Check sheet for the modelled part. Datum: model origin and axes. Units: mm. A direction names the side the tool comes from. Give positions to 0.01 mm unless a question says otherwise; leave off trailing zeros. Loops run counter-clockwise (first coordinate to the right, second up) from the corner with the lowest first, then second, coordinate; pieces in that order, holes last. Notation, with made-up numbers: M -35,-39 L -8,-39 A29 cw -8,-1 Z; hole C 33.25,-19.5 d8. An arc over 180 degrees is marked long. Use one line per item in the form item = value.
from build123d import *

# Parameters (mm, degrees)
F0_R     = 76.2
F3_T     = -6.35
F0_R_2   = 95.25
F4_DEPTH = 12.7
F6_R     = 95.25
F6_R_2   = 76.2
F7_DEPTH = 12.7


with BuildPart() as f2:
    # F2: sweep along a path in F1
    with BuildLine(Plane.XY) as f2_path:
        Line((0, 0), (0, 152.4))
        ThreePointArc((0, 152.4), (44.6369265472, 260.1630734528), (152.4, 304.8))
        Line((152.4, 304.8), (304.8, 304.8))
    # F0 (on Front) → F2 (sweep)
    with BuildSketch(Plane.XZ):
        Circle(F0_R)
    sweep(path=f2_path.line)

    # F3
    f3_openings = [f2.faces().sort_by_distance(p)[0] for p in [
        (0, 0, 0),
        (304.8, 304.8, 0),
    ]]
    offset(amount=F3_T, openings=f3_openings)

    # F0 (on Front) → F4 (join)
    with BuildSketch(Plane.XZ):
        Circle(F0_R_2)
        Circle(F0_R, mode=Mode.SUBTRACT)
    extrude(amount=-F4_DEPTH)

    # F6 (on line) → F7 (join)
    with BuildSketch(Plane.YZ.offset(304.8)):
        with Locations((304.8, 0)):
            Circle(F6_R)
        with Locations((304.8, 0)):
            Circle(F6_R_2, mode=Mode.SUBTRACT)
    extrude(amount=-F7_DEPTH)


solid = f2.part
1) Depth check by flat-ended pin: pin 1 Ø3 at (y, z) = (249, -32.5) entering from -X; pin 2 Ø5 at (y, z) = (101.5, 27) entering from -X; pin 3 Ø12 at (x, z) = (28.5, 31.5) entering from +Y. Enter the tip coordinate at first touch or a pass-through.
Evaluation:
pin_1 = -47.78
pin_2 = -72.15
pin_3 = 341.3
2) Scan lines: line 1 (Z direction, x = 237, y = 304.8); line 2 (X direction, y = 146, z = -17); line 3 (Y direction, x = 264, z = 30). Record each from-to range of solid material in increasing order.
Evaluation:
line_1 = -76.2 to -69.85, 69.85 to 76.2
line_2 = -74.28 to -67.75, 67.75 to 74.28
line_3 = 234.75 to 241.72, 367.88 to 374.85
3) Section check C-C (z = -82). Record the cut outline in (x, y).
Evaluation:
outline = M -48.46,0 L 48.46,0 L 48.46,12.7 L -48.46,12.7 Z; M 292.1,256.34 L 304.8,256.34 L 304.8,353.26 L 292.1,353.26 Z
4) Release check for a two-part mould opening along Y. For faces 4 (the face through (223.23, 232.12, -22.89)), 5 (the face through (-55.431, 77.267, 42.503)), 6 (the face through (-60.47, 83.528, 46.367)) record: pulls with the +Y half, pulls with the -Y half, needs draft (parallel to the pull), parting line crosses it, or undercut.
Evaluation:
face_4 = parting line crosses it
face_5 = needs draft
face_6 = undercut
5) Section check A-A (z = 0). Record the cut outline in (x, y), then the cut area to 3 significant figures.
Evaluation:
outline = M -95.25,0 L -69.85,0 L -69.85,152.4 A222.25 cw 152.4,374.65 L 304.8,374.65 L 304.8,400.05 L 292.1,400.05 L 292.1,381 L 152.4,381 A228.6 ccw -76.2,152.4 L -76.2,12.7 L -95.25,12.7 Z; M 69.85,0 L 95.25,0 L 95.25,12.7 L 76.2,12.7 L 76.2,152.4 A76.2 cw 152.4,228.6 L 292.1,228.6 L 292.1,209.55 L 304.8,209.55 L 304.8,234.95 L 152.4,234.95 A82.55 ccw 69.85,152.4 Z
area = 7,880 mm^2
6) Section check D-D (z = -27.5). Record the cut outline in (x, y), then the cut area to 3 significant figures.
Evaluation:
outline = M -91.19,0 L -64.21,0 L -64.21,152.4 A216.61 cw 152.4,369.01 L 304.8,369.01 L 304.8,395.99 L 292.1,395.99 L 292.1,375.86 L 152.4,375.86 A223.46 ccw -71.06,152.4 L -71.06,12.7 L -91.19,12.7 Z; M 64.21,0 L 91.19,0 L 91.19,12.7 L 71.06,12.7 L 71.06,152.4 A81.34 cw 152.4,233.74 L 292.1,233.74 L 292.1,213.61 L 304.8,213.61 L 304.8,240.59 L 152.4,240.59 A88.19 ccw 64.21,152.4 Z
area = 8,480 mm^2
7) Set-up check for faces 1 (the face through (-75.587, 6.261, -57.958)), 2 (the face through (298.539, 392.787, -36.481)), 3 (the face through (292.1, 262, 64)): record each of +Z, -Z, +X, -X, +Y, -Y from which the full face is reachable in a straight line by a thin tool's end or side.
Evaluation:
face_1 = -Y
face_2 = +X
face_3 = none
8) Section check B-B (x = 193.5). Record the cut outline in (y, z), then the cut area to 3 significant figures.
Evaluation:
outline = C 304.8,0 d152.4; hole C 304.8,0 d139.7
area = 2,910 mm^2
